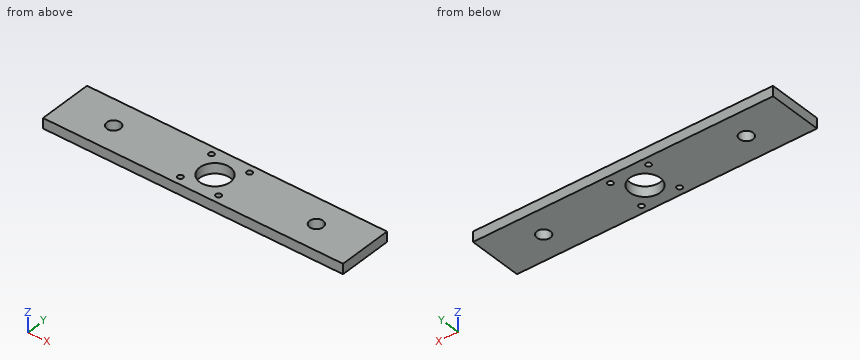
from build123d import *

# Parameters (mm, degrees)
CROQUIS1_W              = 444
CROQUIS1_H              = 80
CROQUIS1_R              = 22.5
CROQUIS1_R_2            = 4
CROQUIS1_R_3            = 10
SALIENTE_EXTRUIR1_DEPTH = 15


with BuildPart() as part:
    # Croquis1 → Saliente-Extruir1 (new body)
    with BuildSketch(Plane.XY):
        Rectangle(CROQUIS1_W, CROQUIS1_H)
        Circle(CROQUIS1_R, mode=Mode.SUBTRACT)
        with Locations((28.25, 28.25)):
            Circle(CROQUIS1_R_2, mode=Mode.SUBTRACT)
        with Locations((-28.25, 28.25)):
            Circle(CROQUIS1_R_2, mode=Mode.SUBTRACT)
        with Locations((28.25, -28.25)):
            Circle(CROQUIS1_R_2, mode=Mode.SUBTRACT)
        with Locations((-28.25, -28.25)):
            Circle(CROQUIS1_R_2, mode=Mode.SUBTRACT)
        with Locations((-150, 0)):
            Circle(CROQUIS1_R_3, mode=Mode.SUBTRACT)
        with Locations((150, 0)):
            Circle(CROQUIS1_R_3, mode=Mode.SUBTRACT)
    extrude(amount=-SALIENTE_EXTRUIR1_DEPTH)


solid = part.part
Can you work these out from the model? Positions are in its coordinate system, mm. Coordinates: 2 decimals unless noted, no trailing zeros. Write each loop counter-clockwise with the first axis right and the second up, starting at its lowest first coordinate (ties: lowest second). Pieces come first, ordered by that corner, then holes.
Q1. For P1, Ø7, axis at x = 28.25, y = -28.25, coming from the +Z side, with a flat end and sliding along its axis, tell me the tip position at first contact or that it passes through.
Results found:
P1: passes through
Q2. Imagine slicing it at A-A, the plane z = -8.75. List the corners of the cut face in (x, y) for me.
Results found:
outline: (-222, -40) - (222, -40) - (222, 40) - (-222, 40) - close; hole circle Ø20 at (-150, 0); hole circle Ø8 at (-28.25, -28.25); hole circle Ø8 at (-28.25, 28.25); hole circle Ø45 at (0, 0); hole circle Ø8 at (28.25, -28.25); hole circle Ø8 at (28.25, 28.25); hole circle Ø20 at (150, 0)
Q3. Imagine slicing it at B-B, the plane x = 150. List the corners of the cut face in (y, z) for me, plus the area to 3 significant figures.
Results found:
outline: (-40, -15) - (-10, -15) - (-10, 0) - (-40, 0) - close; (10, -15) - (40, -15) - (40, 0) - (10, 0) - close
area: 900 mm2
Q4. Please list where these lines run through material, in increasing order: L1, parallel to X at y = -1, z = -5.75; L2, parallel to Y at x = 27.5, z = -13.5; L3, parallel to Y at x = -150, z = -8.
Results found:
L1: x = -222 to -159.95, -140.05 to -22.48, 22.48 to 140.05, 159.95 to 222
L2: y = -40 to -32.18, -24.32 to 24.32, 32.18 to 40
L3: y = -40 to -10, 10 to 40
Q5. Imagine slicing it at D-D, the plane x = 28.25. List the corners of the cut face in (y, z) for me.
Results found:
outline: (-40, -15) - (-32.25, -15) - (-32.25, 0) - (-40, 0) - close; (-24.25, -15) - (24.25, -15) - (24.25, 0) - (-24.25, 0) - close; (32.25, -15) - (40, -15) - (40, 0) - (32.25, 0) - close
Q6. Imagine slicing it at C-C, the plane y = 0. List the corners of the cut face in (x, z) for me, plus the area to 4 significant figures.
Results found:
outline: (-222, -15) - (-160, -15) - (-160, 0) - (-222, 0) - close; (-140, -15) - (-22.5, -15) - (-22.5, 0) - (-140, 0) - close; (22.5, -15) - (140, -15) - (140, 0) - (22.5, 0) - close; (160, -15) - (222, -15) - (222, 0) - (160, 0) - close
area: 5,385 mm2
